from build123d import *

# Parameters (mm, degrees)
SKETCH1_R                            = 65.0875
BOSS_EXTRUDE1_DEPTH                  = 4.7752
SKETCH5_R                            = 12.065
CUT_EXTRUDE2_DEPTH                   = 274.386896239
F_8_32_TAPPED_HOLE1_AT_2_COUNT       = 2
F_8_32_TAPPED_HOLE1_AT_2_PITCH       = 12.7
F_8_32_TAPPED_HOLE1_AT_3_COUNT       = 2
F_8_32_TAPPED_HOLE1_AT_3_PITCH       = 171.45
F_8_32_TAPPED_HOLE1_AT_4_COUNT       = 2
F_8_32_TAPPED_HOLE1_AT_4_PITCH       = 104.89298661
F_8_32_TAPPED_HOLE1_AT_5_COUNT       = 2
F_8_32_TAPPED_HOLE1_AT_5_PITCH       = 112.388811988
F_8_32_TAPPED_HOLE2_AT_2_COUNT       = 2
F_8_32_TAPPED_HOLE2_AT_2_PITCH       = 19.05
CIRPATTERN1_COUNT                    = 2
F_7_0_201_DIAMETER_HOLE1_AT_2_COUNT  = 2
F_7_0_201_DIAMETER_HOLE1_AT_2_PITCH  = 104.778276415
F_7_0_201_DIAMETER_HOLE1_AT_3_COUNT  = 2
F_7_0_201_DIAMETER_HOLE1_AT_3_PITCH  = 186.786089217
F_7_0_201_DIAMETER_HOLE1_AT_4_COUNT  = 2
F_7_0_201_DIAMETER_HOLE1_AT_4_PITCH  = 234.95
F_7_0_201_DIAMETER_HOLE1_AT_5_COUNT  = 2
F_7_0_201_DIAMETER_HOLE1_AT_5_PITCH  = 157.21861372
F_7_0_201_DIAMETER_HOLE1_AT_6_COUNT  = 2
F_7_0_201_DIAMETER_HOLE1_AT_6_PITCH  = 194.790842957
F_7_0_201_DIAMETER_HOLE1_AT_7_COUNT  = 2
F_7_0_201_DIAMETER_HOLE1_AT_7_PITCH  = 345.068605498
F_7_0_201_DIAMETER_HOLE1_AT_8_COUNT  = 2
F_7_0_201_DIAMETER_HOLE1_AT_8_PITCH  = 148.455325494
F_7_0_201_DIAMETER_HOLE1_AT_9_COUNT  = 2
F_7_0_201_DIAMETER_HOLE1_AT_9_PITCH  = 56.772687292
F_7_0_201_DIAMETER_HOLE1_AT_10_COUNT = 2
F_7_0_201_DIAMETER_HOLE1_AT_10_PITCH = 50.8
FILLET1_R                            = 4.7752
CUT_EXTRUDE4_REACH                   = 275.387


with BuildPart() as part:
    # Sketch1 → Boss-Extrude1 (new body)
    with BuildSketch(Plane.XY):
        with BuildLine():
            Line((-63.5, 139.7), (-139.7, 63.5))
            Line((-139.7, 63.5), (-139.7, 12.7))
            Line((-139.7, 12.7), (-71.933056572, -55.066943428))
            ThreePointArc((-71.933056572, -55.066943428), (-70.391368765, -57.374242285), (-69.85, -60.095886856))
            Line((-69.85, -60.095886856), (-69.85, -234.95))
            Line((-69.85, -234.95), (-53.975, -234.95))
            Line((-53.975, -234.95), (139.7, -41.275))
            Line((139.7, -41.275), (139.7, 63.5))
            Line((139.7, 63.5), (63.5, 139.7))
            Line((63.5, 139.7), (-63.5, 139.7))
        make_face()
        Circle(SKETCH1_R, mode=Mode.SUBTRACT)
    extrude(amount=BOSS_EXTRUDE1_DEPTH)

    # Sketch5 → Cut-Extrude2 (cut, through all)
    with BuildSketch(Plane.XY):
        with Locations((117.475, 53.975)):
            Circle(SKETCH5_R)
    extrude(amount=CUT_EXTRUDE2_DEPTH, mode=Mode.SUBTRACT)

    # Sketch6 → #8-32 Tapped Hole1 (revolve, cut)
    with BuildSketch(Plane(origin=(-71.842048969, 49.391408666, 0), x_dir=(0, 1, 0), z_dir=(1, 0, 0))):
        Polygon((0, 0), (0, 4.7752), (2.286, 4.7752), (1.7272, 4.2164), (1.7272, 0.5588), (2.286, 0), align=None)
    f_8_32_tapped_hole1 = revolve(axis=Axis((-71.842048969, 49.391408666, -6.35), (0, 0, 1)), mode=Mode.SUBTRACT)

    # #8-32 Tapped Hole1 at 2: #8-32 Tapped Hole1 ×2
    with Locations(*[Vector(-0.7071067811865428, -0.7071067811865523, 0) * (i * F_8_32_TAPPED_HOLE1_AT_2_PITCH) for i in range(1, F_8_32_TAPPED_HOLE1_AT_2_COUNT)]):
        add(f_8_32_tapped_hole1, mode=Mode.SUBTRACT)

    # #8-32 Tapped Hole1 at 3: #8-32 Tapped Hole1 ×2
    with Locations(*[Vector(0.7071067811865512, -0.7071067811865439, 0) * (i * F_8_32_TAPPED_HOLE1_AT_3_PITCH) for i in range(1, F_8_32_TAPPED_HOLE1_AT_3_COUNT)]):
        add(f_8_32_tapped_hole1, mode=Mode.SUBTRACT)

    # #8-32 Tapped Hole1 at 4: #8-32 Tapped Hole1 ×2
    with Locations(*[Vector(0.09640080542168707, -0.9953425966540617, 0) * (i * F_8_32_TAPPED_HOLE1_AT_4_PITCH) for i in range(1, F_8_32_TAPPED_HOLE1_AT_4_COUNT)]):
        add(f_8_32_tapped_hole1, mode=Mode.SUBTRACT)

    # #8-32 Tapped Hole1 at 5: #8-32 Tapped Hole1 ×2
    with Locations(*[Vector(0.1497391036814564, -0.9887255437322706, 0) * (i * F_8_32_TAPPED_HOLE1_AT_5_PITCH) for i in range(1, F_8_32_TAPPED_HOLE1_AT_5_COUNT)]):
        add(f_8_32_tapped_hole1, mode=Mode.SUBTRACT)

    # Sketch16 → #8-32 Tapped Hole2 (revolve, cut)
    with BuildSketch(Plane(origin=(-18.875314701, 67.922533963, 0), x_dir=(0, 1, 0), z_dir=(1, 0, 0))):
        Polygon((0, 0), (0, 4.7752), (2.286, 4.7752), (1.7272, 4.2164), (1.7272, 0.5588), (2.286, 0), align=None)
    f_8_32_tapped_hole2 = revolve(axis=Axis((-18.875314701, 67.922533963, -6.35), (0, 0, 1)), mode=Mode.SUBTRACT)

    # #8-32 Tapped Hole2 at 2: #8-32 Tapped Hole2 ×2
    with Locations(*[Vector(0.990830168044299, 0.13511320473331287, 0) * (i * F_8_32_TAPPED_HOLE2_AT_2_PITCH) for i in range(1, F_8_32_TAPPED_HOLE2_AT_2_COUNT)]):
        add(f_8_32_tapped_hole2, mode=Mode.SUBTRACT)

    # CirPattern1: #8-32 Tapped Hole2 ×2 about axis
    cirpattern1_axis = Axis((0, 0, 0), (0, 0, 1))
    for i in range(1, CIRPATTERN1_COUNT):
        add(f_8_32_tapped_hole2.rotate(cirpattern1_axis, i * 360 / CIRPATTERN1_COUNT), mode=Mode.SUBTRACT)

    # CirPattern1 copy 1 sketch → CirPattern1 copy 1 (revolve, cut)
    with BuildSketch(Plane(origin=(0, -70.496440513, 0), x_dir=(0, -1, 0), z_dir=(-1, 0, 0))):
        Polygon((0, 0), (0, 4.7752), (2.286, 4.7752), (1.7272, 4.2164), (1.7272, 0.5588), (2.286, 0), align=None)
    revolve(axis=Axis((0, -70.496440513, -6.35), (0, 0, 1)), mode=Mode.SUBTRACT)

    # Sketch9 → #7 (0.201) Diameter Hole1 (revolve, cut)
    with BuildSketch(Plane(origin=(25.4, 133.35, 0), x_dir=(0, 1, 0), z_dir=(1, 0, 0))):
        Polygon((0, 0), (0, 4.7752), (2.6035, 4.7752), (2.5527, 4.652557951), (2.5527, 0.122642049), (2.6035, 0), align=None)
    f_7_0_201_diameter_hole1 = revolve(axis=Axis((25.4, 133.35, -6.35), (0, 0, 1)), mode=Mode.SUBTRACT)

    # #7 (0.201) Diameter Hole1 at 2: #7 (0.201) Diameter Hole1 ×2
    with Locations(*[Vector(0.8558108345517201, -0.5172889090864876, 0) * (i * F_7_0_201_DIAMETER_HOLE1_AT_2_PITCH) for i in range(1, F_7_0_201_DIAMETER_HOLE1_AT_2_COUNT)]):
        add(f_7_0_201_diameter_hole1, mode=Mode.SUBTRACT)

    # #7 (0.201) Diameter Hole1 at 3: #7 (0.201) Diameter Hole1 ×2
    with Locations(*[Vector(-0.8499026917123796, -0.5269396688616753, 0) * (i * F_7_0_201_DIAMETER_HOLE1_AT_3_PITCH) for i in range(1, F_7_0_201_DIAMETER_HOLE1_AT_3_COUNT)]):
        add(f_7_0_201_diameter_hole1, mode=Mode.SUBTRACT)

    # #7 (0.201) Diameter Hole1 at 4: #7 (0.201) Diameter Hole1 ×2
    with Locations(*[Vector(-0.32432432432432445, -0.9459459459459459, 0) * (i * F_7_0_201_DIAMETER_HOLE1_AT_4_PITCH) for i in range(1, F_7_0_201_DIAMETER_HOLE1_AT_4_COUNT)]):
        add(f_7_0_201_diameter_hole1, mode=Mode.SUBTRACT)

    # #7 (0.201) Diameter Hole1 at 5: #7 (0.201) Diameter Hole1 ×2
    with Locations(*[Vector(0.6866235329637165, -0.7270131525498176, 0) * (i * F_7_0_201_DIAMETER_HOLE1_AT_5_PITCH) for i in range(1, F_7_0_201_DIAMETER_HOLE1_AT_5_COUNT)]):
        add(f_7_0_201_diameter_hole1, mode=Mode.SUBTRACT)

    # #7 (0.201) Diameter Hole1 at 6: #7 (0.201) Diameter Hole1 ×2
    with Locations(*[Vector(0.3259906833194041, -0.9453729816262723, 0) * (i * F_7_0_201_DIAMETER_HOLE1_AT_6_PITCH) for i in range(1, F_7_0_201_DIAMETER_HOLE1_AT_6_COUNT)]):
        add(f_7_0_201_diameter_hole1, mode=Mode.SUBTRACT)

    # #7 (0.201) Diameter Hole1 at 7: #7 (0.201) Diameter Hole1 ×2
    with Locations(*[Vector(-0.22082565259779527, -0.9753132989735954, 0) * (i * F_7_0_201_DIAMETER_HOLE1_AT_7_PITCH) for i in range(1, F_7_0_201_DIAMETER_HOLE1_AT_7_COUNT)]):
        add(f_7_0_201_diameter_hole1, mode=Mode.SUBTRACT)

    # #7 (0.201) Diameter Hole1 at 8: #7 (0.201) Diameter Hole1 ×2
    with Locations(*[Vector(-0.9309693618526736, -0.3650973120849093, 0) * (i * F_7_0_201_DIAMETER_HOLE1_AT_8_PITCH) for i in range(1, F_7_0_201_DIAMETER_HOLE1_AT_8_COUNT)]):
        add(f_7_0_201_diameter_hole1, mode=Mode.SUBTRACT)

    # #7 (0.201) Diameter Hole1 at 9: #7 (0.201) Diameter Hole1 ×2
    with Locations(*[Vector(0.9467467942991173, -0.321979048207092, 0) * (i * F_7_0_201_DIAMETER_HOLE1_AT_9_PITCH) for i in range(1, F_7_0_201_DIAMETER_HOLE1_AT_9_COUNT)]):
        add(f_7_0_201_diameter_hole1, mode=Mode.SUBTRACT)

    # #7 (0.201) Diameter Hole1 at 10: #7 (0.201) Diameter Hole1 ×2
    with Locations(*[(-i * F_7_0_201_DIAMETER_HOLE1_AT_10_PITCH, 0, 0) for i in range(1, F_7_0_201_DIAMETER_HOLE1_AT_10_COUNT)]):
        add(f_7_0_201_diameter_hole1, mode=Mode.SUBTRACT)

    # Sketch11 → #10-32 Tapped Hole1 (revolve, cut)
    with BuildSketch(Plane(origin=(42.0624, -103.1875, 0), x_dir=(0, 1, 0), z_dir=(1, 0, 0))):
        Polygon((0, 0), (0, 4.7752), (2.6543, 4.7752), (2.0193, 4.1402), (2.0193, 0.5207), (2.54, 0), align=None)
    revolve(axis=Axis((42.0624, -103.1875, -6.35), (0, 0, 1)), mode=Mode.SUBTRACT)

    # Fillet1
    fillet1_edges = [part.edges().sort_by_distance(p)[0] for p in [
        (-139.7, 63.5, 2.3876),
        (-63.5, 139.7, 2.3876),
        (63.5, 139.7, 2.3876),
        (139.7, 63.5, 2.3876),
        (139.7, -41.275, 2.3876),
    ]]
    fillet(fillet1_edges, radius=FILLET1_R)

    # Sketch13 → Cut-Extrude4 (cut, up to next)
    with BuildSketch(Plane.XY.offset(4.7752), mode=Mode.PRIVATE) as cut_extrude4_sk1:
        with BuildLine():
            Line((3.625876594, 139.7), (9.926476513, 140.251231066))
            Line((9.926476513, 140.251231066), (9.926476513, 142.770744163))
            Line((9.926476513, 142.770744163), (-16.276476513, 142.770744163))
            Line((-16.276476513, 142.770744163), (-16.276476513, 140.251231066))
            Line((-16.276476513, 140.251231066), (-9.975876594, 139.7))
            ThreePointArc((-9.975876594, 139.7), (-9.686584819, 139.577074227), (-9.525, 139.30746187))
            ThreePointArc((-9.525, 139.30746187), (-8.667649526, 137.945233031), (-7.148271788, 137.414))
            Line((-7.148271788, 137.414), (0.798271788, 137.414))
            ThreePointArc((0.798271788, 137.414), (2.317649526, 137.945233031), (3.175, 139.30746187))
            ThreePointArc((3.175, 139.30746187), (3.336584819, 139.577074227), (3.625876594, 139.7))
        make_face()
    cut_extrude4_tool1 = extrude(cut_extrude4_sk1.sketch, amount=-CUT_EXTRUDE4_REACH, mode=Mode.PRIVATE) & part.part
    add(cut_extrude4_tool1.solids().sort_by_distance((-3.175, 140.603778, 4.7752))[0], mode=Mode.SUBTRACT)


solid = part.part
Input: part model. Units: mm. Frame: model coordinates. Give positions to 0.01 mm unless a question says otherwise; leave off trailing zeros. Order: outer loops, then holes, each group sorted by start corner. A loop starts at its lowest first (then second) coordinate and runs counter-clockwise, first axis right, second up.
Q1. Contact query for flat-ended pins moving along their axis: pin 1 Ø1.4 at (y, z) = (-117, 3) entering from -X; pin 2 Ø4 at (x, y) = (-18.88, 67.92) entering from -Z. Output: stop coordinate, or through.
Checked values:
pin 1: stops at x = -69.85
pin 2: stops at z = 0.28
Q2. Draft query along X for faces 1 (the flat face through (-106, -21, 2)), 2 (the flat face through (102.1, 101.1, 2.4)), 3 (the cylindrical face through (-51.651, -39.605, 2.354)). Return one class per face: +X half, -X half, draft (parallel to the pull), parting line (faces both ways), or undercut.
Checked values:
face 1: -X half
face 2: +X half
face 3: undercut
Q3. Ray query, probe 1 along Y at (x, z) = (19.5, 1.6) (3 decimals); probe 2 along Y at (x, z) = (48.5, 1.55) (3 decimals); probe 3 along Y at (x, z) = (-50.8, 2) (3 decimals). Return the intervals inside material, ascending.
Checked values:
probe 1: y = -161.475 to -69.533, -66.312 to -62.098, 62.098 to 139.7
probe 2: y = -132.475 to -73.321, -70.363 to -43.407, 43.407 to 139.7
probe 3: y = -231.775 to -205.753, -200.647 to -91.453, -86.347 to -40.691, 40.691 to 139.7
Q4. Section B-B on z = 2.1. State how many separate pieces and enclosed holes the cut face has, and give its area (3 significant figures).
Checked values:
separate pieces: 1
enclosed holes: 22
area: 51,200 mm2
Q5. Section C-C on y = -162. Output: boundary loops of the cut face in (x, z) (3 decimals), and give its area (3 significant figures).
Checked values:
outline: (-69.85, 0) - (18.975, 0) - (18.975, 4.775) - (-69.85, 4.775) - close
area: 424 mm2
Q6. Section A-A on y = 0. Output: boundary loops of the cut face in (x, z), and give its area (3 significant figures).
Checked values:
outline: (-127, 0) - (-65.09, 0) - (-65.09, 4.78) - (-127, 4.78) - close; (65.09, 0) - (139.7, 0) - (139.7, 4.78) - (65.09, 4.78) - close
area: 652 mm2
